```python
from build123d import *

# Parameters (mm, degrees)
BOSS_EXTRUDE1_DEPTH = 63.5
CUT_EXTRUDE2_REACH  = 82.274
CUT_EXTRUDE2_START  = -3.81
SKETCH2_W           = 68.58
SKETCH2_H           = 55.88


with BuildPart() as part:
    # Sketch1 → Boss-Extrude1 (new body)
    with BuildSketch(Plane.XY):
        with BuildLine():
            Line((-38.1, 9.525), (-38.1, -9.525))
            Line((-38.1, -9.525), (38.1, -9.525))
            Line((38.1, -9.525), (38.1, 9.525))
            Line((38.1, 9.525), (30.7975, 9.525))
            Line((30.7975, 9.525), (30.7975, -1.905))
            ThreePointArc((30.7975, -1.905), (28.8925, -3.81), (26.9875, -1.905))
            Line((26.9875, -1.905), (26.9875, 9.525))
            Line((26.9875, 9.525), (22.5425, 9.525))
            Line((22.5425, 9.525), (22.5425, -1.905))
            ThreePointArc((22.5425, -1.905), (20.6375, -3.81), (18.7325, -1.905))
            Line((18.7325, -1.905), (18.7325, 9.525))
            Line((18.7325, 9.525), (14.2875, 9.525))
            Line((14.2875, 9.525), (14.2875, -1.905))
            ThreePointArc((14.2875, -1.905), (12.3825, -3.81), (10.4775, -1.905))
            Line((10.4775, -1.905), (10.4775, 9.525))
            Line((10.4775, 9.525), (6.0325, 9.525))
            Line((6.0325, 9.525), (6.0325, -1.905))
            ThreePointArc((6.0325, -1.905), (4.1275, -3.81), (2.2225, -1.905))
            Line((2.2225, -1.905), (2.2225, 9.525))
            Line((2.2225, 9.525), (-2.2225, 9.525))
            Line((-2.2225, 9.525), (-2.2225, -1.905))
            ThreePointArc((-2.2225, -1.905), (-4.1275, -3.81), (-6.0325, -1.905))
            Line((-6.0325, -1.905), (-6.0325, 9.525))
            Line((-6.0325, 9.525), (-10.4775, 9.525))
            Line((-10.4775, 9.525), (-10.4775, -1.905))
            ThreePointArc((-10.4775, -1.905), (-12.3825, -3.81), (-14.2875, -1.905))
            Line((-14.2875, -1.905), (-14.2875, 9.525))
            Line((-14.2875, 9.525), (-18.7325, 9.525))
            Line((-18.7325, 9.525), (-18.7325, -1.905))
            ThreePointArc((-18.7325, -1.905), (-20.6375, -3.81), (-22.5425, -1.905))
            Line((-22.5425, -1.905), (-22.5425, 9.525))
            Line((-22.5425, 9.525), (-26.9875, 9.525))
            Line((-26.9875, 9.525), (-26.9875, -1.905))
            ThreePointArc((-26.9875, -1.905), (-28.8925, -3.81), (-30.7975, -1.905))
            Line((-30.7975, -1.905), (-30.7975, 9.525))
            Line((-30.7975, 9.525), (-38.1, 9.525))
        make_face()
    extrude(amount=BOSS_EXTRUDE1_DEPTH)

    # Sketch2 → Cut-Extrude2 (cut, up to next)
    with BuildSketch(Plane.XZ.offset(9.525).offset(CUT_EXTRUDE2_START), mode=Mode.PRIVATE) as cut_extrude2_sk1:
        with Locations((0, 31.75)):
            Rectangle(SKETCH2_W, SKETCH2_H)
    cut_extrude2_tool1 = extrude(cut_extrude2_sk1.sketch, amount=-CUT_EXTRUDE2_REACH, mode=Mode.PRIVATE) & part.part
    add(cut_extrude2_tool1.solids().sort_by_distance((0, -5.715, 31.75))[0], mode=Mode.SUBTRACT)


solid = part.part
```
Model file for the job. Use its own axes, mm. A direction names the side the tool comes from. Coordinates: 2 decimals unless noted, no trailing zeros. Loops run counter-clockwise (first coordinate to the right, second up) from the corner with the lowest first, then second, coordinate; pieces in that order, holes last. Notation, with made-up numbers: (31.25, 70) -> (86.25, 70) arc R9 ccw to (86.25, 86) -> close; hole circle Ø4 at (-28.5, 46). An arc over 180 degrees is marked (long way). Answer as a JSON object with one key per item and string values.
Q1. Cut at A-A (x = -32). List the corners of the cut face in (y, z) (3 decimals).
Report:
{"outline": "(-9.525, 0) -> (9.525, 0) -> (9.525, 3.81) -> (-5.715, 3.81) -> (-5.715, 59.69) -> (9.525, 59.69) -> (9.525, 63.5) -> (-9.525, 63.5) -> close"}
Q2. 3-axis set-ups, long thin cutter, end or side, ignore diameter. For faces 1 (the flat face through (-38.1, 0, 31)), 2 (the flat face through (-2.222, 4, 62)), 3 (the flat face through (-8, 2, 3.81)): which of +Z, -Z, +X, -X, +Y, -Y reach the whole face in a straight line?
Report:
{"face 1": "+Z, -Z, -X, +Y, -Y", "face 2": "+Z, -Z, +Y", "face 3": "+Y"}
Q3. Cut at C-C (y = 5.5). State how many separate pieces and enclosed holes the cut face has, and give its area (3 significant figures).
Report:
{"separate pieces": "16", "enclosed holes": "0", "area": "774 mm2"}
Q4. Cut at B-B (z = 27). List the corners of the cut face in (x, y) (3 decimals).
Report:
{"outline": "(-38.1, -9.525) -> (38.1, -9.525) -> (38.1, 9.525) -> (34.29, 9.525) -> (34.29, -5.715) -> (-34.29, -5.715) -> (-34.29, 9.525) -> (-38.1, 9.525) -> close"}
Q5. Probe probe 1 along Z at (x, y) = (-12.5, -4); probe 2 along X at (y, z) = (1.25, 44.5); probe 3 along Y at (x, z) = (-23, 43) (3 decimals). List the from-to ranges inside material, lowest first.
Report:
{"probe 1": "z = 0 to 3.81, 59.69 to 63.5", "probe 2": "x = -38.1 to -34.29, 34.29 to 38.1", "probe 3": "y = -9.525 to -5.715"}
Q6. Flat gauge pin, fed straight in: P1, Ø12, axis at x = 0, z = 25.5, coming from the +Y side (3 decimals). Where does the tip first touch, or does it go through?
Report:
{"P1": "stops at y = -5.715"}
Q7. Pull direction Z, two halves, no side cores. Call faces 4 (the flat face through (14.288, 4, 2)), 5 (the flat face through (34.29, 2, 31)): released by +Z, released by -Z, zero draft, split by the parting line, or undercut.
Report:
{"face 4": "zero draft", "face 5": "undercut"}
